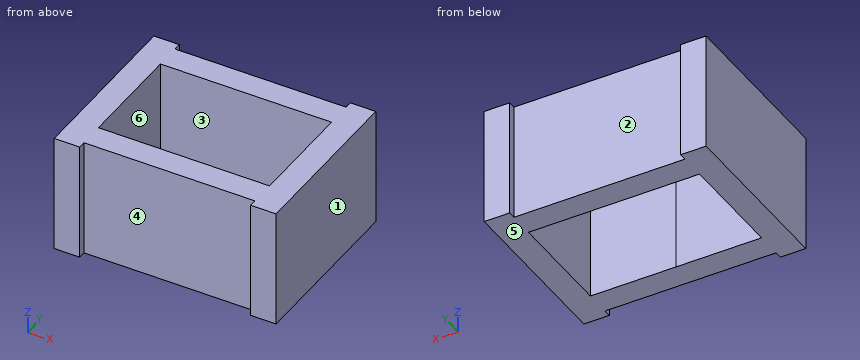
Autodesk Inventor part; units mm, degrees
ref_plane "YZ Plane" through (0, 0, 0) normal (1, 0, 0) x (0, 1, 0)
ref_plane "XZ Plane" through (0, 0, 0) normal (0, 1, 0) x (-1, 0, 0)
ref_plane "XY Plane" through (0, 0, 0) normal (0, 0, 1) x (1, 0, 0)
sketch "Sketch1" plane through (0, 0, 0) normal (0, 0, 1) x (1, 0, 0)
  line L0 (0, 0) -> (166.6875, 0)
  line L1 (166.6875, 0) -> (166.6875, 130.175)
  line L2 (166.6875, 130.175) -> (0, 130.175)
  line L3 (0, 130.175) -> (0, 0)
  dimension "d0" = 166.6875
  dimension "d1" = 130.175
extrude "Extrusion1" add sketch "Sketch1" along normal blind 88.9
sketch "Sketch3" plane through (0, 0, 0) normal (0, 0, -1) x (-1, 0, 0)
  line L0 (-166.6875, 0) -> (-166.6875, 130.175) construction
  line L1 (0, 0) -> (-166.6875, 0)
  line L2 (0, 130.175) -> (0, 0) construction
  line L3 (-166.6875, 130.175) -> (0, 130.175) construction
  line L4 (-166.6875, 0) -> (-147.6375, 0) construction
  line L5 (-147.6375, 0) -> (-147.6375, 5.5563)
  line L6 (0, 0) -> (-166.6875, 0) construction
  line L7 (-83.3438, 0) -> (-83.3438, 30.0341) construction
  line L8 (-166.6875, 0) -> (0, 0) construction
  line L9 (0, 0) -> (-19.05, 0) construction
  line L10 (-19.05, 0) -> (-19.05, 5.5563)
  line L11 (-166.6875, 0) -> (0, 0) construction
  line L12 (-19.05, 5.5563) -> (-147.6375, 5.5563)
  line L13 (-147.6375, 5.5563) -> (-19.05, 5.5563)
  line L14 (-19.05, 5.5563) -> (-19.05, 0)
  line L15 (-19.05, 0) -> (-147.6375, 0)
  line L16 (-147.6375, 0) -> (-147.6375, 5.5563)
  line L17 (-166.6875, 65.0875) -> (-112.8864, 65.0875) construction
  line L18 (-147.6375, 130.175) -> (-147.6375, 124.6187)
  line L19 (-19.05, 130.175) -> (-19.05, 124.6187)
  line L20 (-19.05, 124.6187) -> (-147.6375, 124.6187)
  line L21 (-147.6375, 124.6187) -> (-19.05, 124.6187)
  line L22 (-19.05, 124.6187) -> (-19.05, 130.175)
  line L23 (-19.05, 130.175) -> (-147.6375, 130.175)
  line L24 (-147.6375, 130.175) -> (-147.6375, 124.6187)
  point P0 (-83.3438, 130.175)
extrude "Extrusion2" cut sketch "Sketch3" against normal through all
sketch "Sketch4" plane through (0, 0, 0) normal (0, 0, -1) x (-1, 0, 0)
  line L0 (-147.6375, 124.6187) -> (-147.6375, 130.175)
  line L1 (-166.6875, 130.175) -> (-147.6375, 130.175)
  line L2 (-166.6875, 0) -> (-166.6875, 130.175)
  line L3 (-147.6375, 0) -> (-166.6875, 0)
  line L4 (-147.6375, 0) -> (-147.6375, 5.5563)
  line L5 (-147.6375, 5.5563) -> (-19.05, 5.5563)
  line L6 (-19.05, 5.5563) -> (-19.05, 0)
  line L7 (0, 0) -> (-19.05, 0)
  line L8 (0, 130.175) -> (0, 0)
  line L9 (-19.05, 130.175) -> (0, 130.175)
  line L10 (-19.05, 130.175) -> (-19.05, 124.6187)
  line L11 (-19.05, 124.6187) -> (-147.6375, 124.6187)
  line L12 (-147.6375, 124.6187) -> (-147.6375, 5.5563) construction
  line L13 (-19.05, 5.5563) -> (-19.05, 124.6187) construction
  line L14 (-19.05, 124.6187) -> (-147.6375, 124.6187) construction
  line L15 (-83.3438, 124.6187) -> (-83.3438, 105.5687) construction
  line L16 (-83.3438, 105.5687) -> (-19.05, 105.5687)
  line L17 (-83.3438, 105.5687) -> (-147.6375, 105.5687)
  line L18 (-147.6375, 65.0875) -> (-19.05, 65.0875) construction
  line L19 (-83.3438, 24.6062) -> (-19.05, 24.6063)
  line L20 (-83.3438, 24.6062) -> (-147.6375, 24.6062)
  line L21 (-147.6375, 105.5687) -> (-147.6375, 24.6062)
  line L22 (-19.05, 24.6063) -> (-19.05, 105.5687)
  dimension "d8" = 19.05
extrude "Extrusion3" cut sketch "Sketch4" against normal through all contours L16 L22 L19 L20 L21 L17
properties part number "Magnet"
The model under review builds one solid part; all positions refer to its coordinate system, in mm. Face numbers are marked on the shaded views. A direction names the side the tool comes from. Give positions to 0.01 mm unless a question says otherwise; leave off trailing zeros. Order: outer loops, then holes, each group sorted by start corner. A loop starts at its lowest first (then second) coordinate and runs counter-clockwise, first axis right, second up. Notation, with made-up numbers: M -18.5,-12 L 10.5,-12 A10 ccw 10.5,-7 Z; hole C 88.5,32 d8. An arc over 180 degrees is marked long. Answer in a Markdown table with one row per item. Add a question column.
1. Machinability: for the marked faces 1, 2 and 3, which of the approach directions +Z, -Z, +X, -X, +Y, -Y give a long, thin tool a straight path to every point of the face, cutting with its end or side? Answer none if there is none.
2. For pin 1 Ø10 at (x, z) = (76, 72.5) entering from -Y; pin 2 Ø5 at (x, z) = (86, 50) entering from +Y, all flat-tipped, find the tip position at first contact; note any pin that passes through.
3. Add section A-A on y = 54.5. State the section outline as (x, z) points.
4. To check wall thickness, follow line 1 along Y through (x, z) = (132, 77); line 2 along X through (y, z) = (38, 46). State the ranges of each line that lie inside material, in increasing order.
5. Mouldability with a two-part tool opening along Y and no side actions: class the marked faces 4, 5 and 6 as released by +Y, released by -Y, zero draft, split by the parting line, or undercut.
6. Add section C-C on x = 21. State the section outline as (y, z) points, plus the area to 3 significant figures.
The answers:
| question | item | result |
|---|---|---|
| 1 | face 1 | +Z, -Z, +X, +Y, -Y |
| 1 | face 2 | +Z, -Z, +Y |
| 1 | face 3 | +Z, -Z |
| 2 | pin 1 | y = 5.56 |
| 2 | pin 2 | y = 124.62 |
| 3 | outline | M 0,0 L 19.05,0 L 19.05,88.9 L 0,88.9 Z; M 147.64,0 L 166.69,0 L 166.69,88.9 L 147.64,88.9 Z |
| 4 | line 1 | 5.56 to 24.61, 105.57 to 124.62 |
| 4 | line 2 | 0 to 19.05, 147.64 to 166.69 |
| 5 | face 4 | released by -Y |
| 5 | face 5 | zero draft |
| 5 | face 6 | undercut |
| 6 | outline | M 5.56,0 L 24.61,0 L 24.61,88.9 L 5.56,88.9 Z; M 105.57,0 L 124.62,0 L 124.62,88.9 L 105.57,88.9 Z |
| 6 | area | 3,390 mm2 |
